from build123d import *

# Parameters (mm, degrees)
SKETCH1_R               = 12
BOSS_EXTRUDE1_DEPTH     = 4
SKETCH3_W               = 3
SKETCH3_H               = 3.312885388
SKETCH6_R               = 8.5
BOSS_EXTRUDE2_DEPTH     = 6
CUT_EXTRUDE1_DEPTH      = 23
CUT_EXTRUDE1_DEPTH_BACK = 23
SKETCH7_R               = 5
CUT_EXTRUDE2_DEPTH      = 20.697715604
CUT_EXTRUDE2_DEPTH_BACK = 20.697715604
SKETCH8_R               = 1.5


with BuildPart() as part:
    # Sketch1 → Boss-Extrude1 (new, symmetric)
    with BuildSketch(Plane.XY):
        Circle(SKETCH1_R)
    extrude(amount=BOSS_EXTRUDE1_DEPTH, both=True)

    # Sketch3 → Cut-Revolve2 (revolve, cut)
    with BuildSketch(Plane(origin=(0, 0, 0), x_dir=(0, 0, -1), z_dir=(1, 0, 0)), mode=Mode.PRIVATE) as cut_revolve2_sk:
        with Locations((0, 11.656442694)):
            Rectangle(SKETCH3_W, SKETCH3_H)
    revolve(cut_revolve2_sk.sketch.rotate(Axis((0, 0, 0), (0, 0, 1)), 90), axis=Axis((0, 0, 0), (0, 0, 1)), mode=Mode.SUBTRACT)

    # Sketch6 → Boss-Extrude2 (add)
    with BuildSketch(Plane.XY.offset(4)):
        with Locations(Location((0, -3.5, 0), (0, 0, 270))):
            Circle(SKETCH6_R)
    extrude(amount=BOSS_EXTRUDE2_DEPTH)

    # Sketch7 → Cut-Extrude1 (cut, two sides: drawn at the far end of the back side and taken through both)
    with BuildSketch(Plane.XY.offset(10).offset(-CUT_EXTRUDE1_DEPTH_BACK)):
        with Locations((0, -3.5)):
            Circle(SKETCH7_R)
    extrude(amount=CUT_EXTRUDE1_DEPTH + CUT_EXTRUDE1_DEPTH_BACK, mode=Mode.SUBTRACT)

    # Sketch8 → Cut-Extrude2 (cut, two sides: drawn at the far end of the back side and taken through both)
    with BuildSketch(Plane(origin=(0, 0, 0), x_dir=(1, 0, 0), z_dir=(0, 1, 0)).offset(-CUT_EXTRUDE2_DEPTH_BACK)):
        with Locations(Location((0, -7, 0), (0, 0, 270))):
            Circle(SKETCH8_R)
    extrude(amount=CUT_EXTRUDE2_DEPTH + CUT_EXTRUDE2_DEPTH_BACK, mode=Mode.SUBTRACT)


solid = part.part
Model file for the job. Use its own axes, mm. A direction names the side the tool comes from. Give positions to 0.01 mm unless a question says otherwise; leave off trailing zeros. Order: outer loops, then holes, each group sorted by start corner. A loop starts at its lowest first (then second) coordinate and runs counter-clockwise, first axis right, second up. Notation, with made-up numbers: (64, -5.75) - (80, -5.75) arc R34 ccw to (80, 28.25) - close; hole circle Ø8 at (23.5, -4). An arc over 180 degrees is marked (long way). One line per item, written item: value.
Item 1: Two-plate mould, pull along Z, no slides. Class faces 1 (the flat face through (0, 6, 4)), 2 (the cylindrical face through (0.07, 3.11, 5.5)), 3 (the flat face through (0, 3, -4)): released by +Z, released by -Z, zero draft, split by the parting line, or undercut.
Response values:
face 1: released by +Z
face 2: undercut
face 3: released by -Z
Item 2: Slice it at A-A (y = 0). List the corners of the cut face in (x, z), then the cut area to 3 significant figures.
Response values:
outline: (-12, -4) - (-3.57, -4) - (-3.57, 10) - (-7.75, 10) - (-7.75, 4) - (-12, 4) - (-12, 1.5) - (-10, 1.5) - (-10, -1.5) - (-12, -1.5) - close; (3.57, -4) - (12, -4) - (12, -1.5) - (10, -1.5) - (10, 1.5) - (12, 1.5) - (12, 4) - (7.75, 4) - (7.75, 10) - (3.57, 10) - close
area: 173 mm2
Item 3: Slice it at B-B (x = 4.5). List the corners of the cut face in (y, z).
Response values:
outline: (-11.12, -4) - (-5.68, -4) - (-5.68, 10) - (-10.71, 10) - (-10.71, 4) - (-11.12, 4) - (-11.12, 1.5) - (-8.93, 1.5) - (-8.93, -1.5) - (-11.12, -1.5) - close; (-1.32, -4) - (11.12, -4) - (11.12, -1.5) - (8.93, -1.5) - (8.93, 1.5) - (11.12, 1.5) - (11.12, 4) - (3.71, 4) - (3.71, 10) - (-1.32, 10) - close
Item 4: Tool access for faces 4 (the flat face through (-5, -9, -1.5)), 5 (the flat face through (-4, -7, 10)), 6 (the cylindrical face through (2.55, -11.61, 6.96)): list every direction of +Z, -Z, +X, -X, +Y, -Y with a clear straight run to the whole face (end or side of a thin tool).
Response values:
face 4: none
face 5: +Z, +X, -X, +Y, -Y
face 6: +Z
Item 5: Slice it at C-C (z = -2.5). List the corners of the cut face in (x, y).
Response values:
outline: circle Ø24 at (0, 0); hole circle Ø10 at (0, -3.5)
Item 6: Pin check, flat tips, straight feed: pin 1 Ø1.5 at (x, y) = (4, 6.5) entering from +Z; pin 2 Ø3.5 at (x, z) = (0, 7) entering from +Y; pin 3 Ø8 at (y, z) = (-9.5, 7.5) entering from -X. Stop position of each tip, or through.
Response values:
pin 1: z = 4
pin 2: y = 5
pin 3: x = -9.32
Item 7: Slice it at D-D (y = 2.5). List the corners of the cut face in (x, z), then the cut area to 3 significant figures.
Response values:
outline: (-11.74, -4) - (11.74, -4) - (11.74, -1.5) - (9.68, -1.5) - (9.68, 1.5) - (11.74, 1.5) - (11.74, 4) - (6.02, 4) - (6.02, 10) - (-6.02, 10) - (-6.02, 4) - (-11.74, 4) - (-11.74, 1.5) - (-9.68, 1.5) - (-9.68, -1.5) - (-11.74, -1.5) - close; hole circle Ø3 at (0, 7)
area: 241 mm2
Item 8: Wall check: line 1 (Y direction, x = 0, z = 2.25); line 2 (Z direction, x = 6, y = 9.5); line 3 (Z direction, x = 0, y = 3.4). Give the ranges that are in metal, low to high.
Response values:
line 1: -12 to -8.5, 1.5 to 12
line 2: -4 to -1.5, 1.5 to 4
line 3: -4 to 5.5, 8.5 to 10
